Geometry: final body of the model. Coordinates: model frame, mm. Face numbers are marked on the shaded views. Give positions to 0.01 mm unless a question says otherwise; leave off trailing zeros. Write each loop counter-clockwise with the first axis right and the second up, starting at its lowest first coordinate (ties: lowest second). Pieces come first, ordered by that corner, then holes.
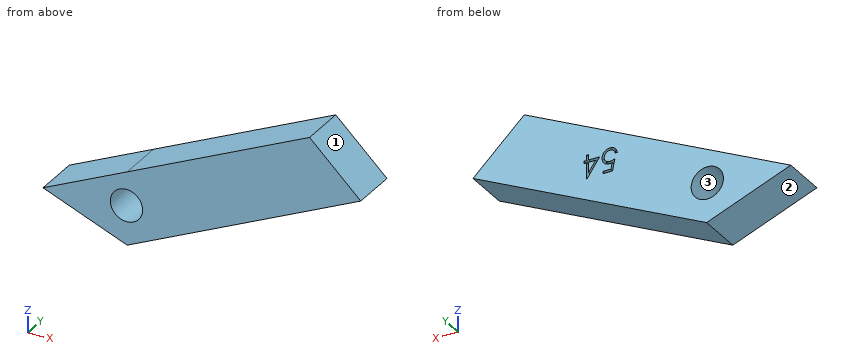
```python
from build123d import *

# Parameters (mm, degrees)
SKETCH1_R           = 2.2
BOSS_EXTRUDE1_DEPTH = 6.2
CUT_EXTRUDE1_DEPTH  = 1


with BuildPart() as part:
    # Sketch1 → Boss-Extrude1 (new body)
    with BuildSketch(Plane(origin=(0, 0, 0), x_dir=(-1, 0, 0), z_dir=(0, 1, 0))):
        Polygon((-127.443880814, 98.339887686), (-134.435779681, 91.672540756), (-102.538529649, 76.502840404), (-91.051660388, 81.032468444), (-102.547087364, 86.499465833), align=None)
        with Locations((-102.448365494, 81.883499702)):
            Circle(SKETCH1_R, mode=Mode.SUBTRACT)
    extrude(amount=BOSS_EXTRUDE1_DEPTH)

    # Sketch2 → Cut-Extrude1 (cut)
    with BuildSketch(Plane(origin=(0, 6.2, 0), x_dir=(1, 0, 0), z_dir=(0, 1, 0))):
        with BuildLine():
            Line((116.688123147, -87.22045081), (116.688123147, -87.546091836))
            Line((116.688123147, -87.546091836), (115.608165214, -87.546091836))
            Line((115.608165214, -87.546091836), (115.437076472, -88.381182982))
            add(Edge.make_bspline(
                [(115.437076472, -88.381182982), (115.470691444, -88.371902664), (115.535815135, -88.353923515), (115.631935866, -88.333961138), (115.723187365, -88.321927485), (115.782401451, -88.320284368), (115.811054838, -88.319489272)],
                knots=[0, 0, 0, 0, 0.000104595, 0.000202637, 0.000294305, 0.000380252, 0.000380252, 0.000380252, 0.000380252], degree=3))
            add(Edge.make_bspline(
                [(115.811054838, -88.319489272), (115.846509373, -88.320256656), (115.916221848, -88.321765526), (116.018220035, -88.336254275), (116.115586303, -88.359059769), (116.208117024, -88.3909191), (116.295983381, -88.431658643), (116.378376955, -88.482549303), (116.45653449, -88.541997397), (116.529053843, -88.610346086), (116.594843751, -88.685567839), (116.652688613, -88.766446764), (116.70182182, -88.852196858), (116.741337648, -88.94363741), (116.772892008, -89.039757499), (116.793894175, -89.141568485), (116.807879332, -89.248110708), (116.809441783, -89.320958425), (116.810238532, -89.358106059)],
                knots=[0, 0, 0, 0, 0.000106308, 0.000209029, 0.000308378, 0.000405929, 0.000502102, 0.000598312, 0.00069588, 0.000796219, 0.000896736, 0.000995218, 0.001094066, 0.001192613, 0.001293582, 0.001396995, 0.001504047, 0.001615439, 0.001615439, 0.001615439, 0.001615439], degree=3))
            add(Edge.make_bspline(
                [(116.810238532, -89.358106059), (116.809635213, -89.383979787), (116.80843673, -89.435377583), (116.802342011, -89.511708394), (116.790607469, -89.586423249), (116.774852462, -89.659532062), (116.754403269, -89.730896421), (116.729648198, -89.800720593), (116.69935323, -89.868569986), (116.66612334, -89.935086594), (116.628706892, -89.998766669), (116.587179246, -90.058319678), (116.543304836, -90.11463899), (116.496095865, -90.167120591), (116.445113534, -90.215419615), (116.390975278, -90.259822698), (116.334113097, -90.301080762), (116.27364727, -90.337519054), (116.210925161, -90.371049735), (116.145040992, -90.398557516), (116.0774945, -90.423150638), (116.007313506, -90.442753566), (115.934656976, -90.458113812), (115.859405144, -90.4685465), (115.781952679, -90.476145125), (115.729451774, -90.476620792), (115.702931841, -90.476861067)],
                knots=[0, 0, 0, 0, 7.7636e-05, 0.000154223, 0.000229512, 0.000304362, 0.000378447, 0.000452077, 0.000526407, 0.000601214, 0.00067506, 0.000747747, 0.00081887, 0.000889121, 0.000959302, 0.001029336, 0.001099058, 0.00116985, 0.001240974, 0.00131221, 0.00138383, 0.001456517, 0.001530612, 0.001606437, 0.001684346, 0.001763871, 0.001763871, 0.001763871, 0.001763871], degree=3))
            add(Edge.make_bspline(
                [(115.702931841, -90.476861067), (115.671295977, -90.476234378), (115.609056152, -90.475001442), (115.517869638, -90.462103245), (115.430135674, -90.443630263), (115.346560511, -90.41583879), (115.26639515, -90.38101603), (115.190718827, -90.337004931), (115.117597873, -90.28713103), (115.050004812, -90.228275281), (114.987270337, -90.163944627), (114.93111229, -90.094133052), (114.88109826, -90.019992773), (114.83802916, -89.941163733), (114.80129167, -89.857853066), (114.77243093, -89.769748629), (114.749136994, -89.677310768), (114.73928232, -89.613671513), (114.734276993, -89.581348246)],
                knots=[0, 0, 0, 0, 9.4843e-05, 0.000186593, 0.000275792, 0.000363484, 0.000450342, 0.000537514, 0.000625728, 0.000715478, 0.000805885, 0.000894984, 0.00098389, 0.001073836, 0.001164117, 0.001256635, 0.001351658, 0.001449737, 0.001449737, 0.001449737, 0.001449737], degree=3))
            Line((114.734276993, -89.581348246), (115.019212891, -89.581348246))
            add(Edge.make_bspline(
                [(115.019212891, -89.581348246), (115.026223796, -89.611625457), (115.039699146, -89.669819936), (115.069277218, -89.751581939), (115.105441262, -89.824442949), (115.148443778, -89.889366785), (115.199742735, -89.945980661), (115.258280145, -89.996433282), (115.323909866, -90.041949292), (115.396838009, -90.079888516), (115.473775589, -90.112245171), (115.554300129, -90.133791352), (115.636219072, -90.148941447), (115.691625879, -90.150457973), (115.719468299, -90.151220041)],
                knots=[0, 0, 0, 0, 9.3172e-05, 0.000179081, 0.000260145, 0.000336703, 0.000411917, 0.000488562, 0.000568128, 0.000650923, 0.00073478, 0.000817953, 0.000900557, 0.000983994, 0.000983994, 0.000983994, 0.000983994], degree=3))
            add(Edge.make_bspline(
                [(115.719468299, -90.151220041), (115.746644888, -90.150475478), (115.800155814, -90.149009428), (115.878906143, -90.137725467), (115.954936393, -90.120346813), (116.027496353, -90.094339159), (116.097855749, -90.062730021), (116.164234813, -90.02216706), (116.228553851, -89.975485472), (116.288813658, -89.922003386), (116.34400373, -89.863066591), (116.392768211, -89.80004067), (116.433387268, -89.732806102), (116.467617496, -89.662526885), (116.493610131, -89.588432765), (116.512153021, -89.510870985), (116.52304151, -89.429649967), (116.524539366, -89.374251379), (116.525302634, -89.346021724)],
                knots=[0, 0, 0, 0, 8.15e-05, 0.000160473, 0.000238226, 0.000315066, 0.000391338, 0.000469218, 0.000547964, 0.000629516, 0.000710512, 0.000789892, 0.000868102, 0.000945761, 0.001024012, 0.00110315, 0.001184644, 0.001269321, 0.001269321, 0.001269321, 0.001269321], degree=3))
            add(Edge.make_bspline(
                [(116.525302634, -89.346021724), (116.524705299, -89.320553006), (116.523536101, -89.270701615), (116.513983369, -89.19776805), (116.497367259, -89.128758933), (116.474304168, -89.06334102), (116.445022043, -89.001452612), (116.409238602, -88.943029836), (116.366282306, -88.888842716), (116.317213235, -88.838865899), (116.263457727, -88.792742334), (116.204090903, -88.753423056), (116.140355112, -88.720345073), (116.073018261, -88.691799103), (116.000478675, -88.671296999), (115.924172873, -88.655904703), (115.843276859, -88.647000766), (115.787967735, -88.645765339), (115.75953741, -88.645130297)],
                knots=[0, 0, 0, 0, 7.6388e-05, 0.000149519, 0.000220172, 0.000288967, 0.000357247, 0.000425206, 0.000494043, 0.000564207, 0.000635056, 0.000706145, 0.000777268, 0.000850264, 0.000925136, 0.001002969, 0.001083601, 0.001168886, 0.001168886, 0.001168886, 0.001168886], degree=3))
            add(Edge.make_bspline(
                [(115.75953741, -88.645130297), (115.734927596, -88.645656977), (115.684114573, -88.646744435), (115.606170295, -88.654751329), (115.524262803, -88.667668403), (115.438706082, -88.685435928), (115.349243193, -88.708686976), (115.256062929, -88.736549416), (115.158969373, -88.769861515), (115.093548295, -88.795018594), (115.059918019, -88.80795081)],
                knots=[0, 0, 0, 0, 7.3822e-05, 0.000152423, 0.000234822, 0.000322511, 0.00041445, 0.000512043, 0.000614219, 0.000722306, 0.000722306, 0.000722306, 0.000722306], degree=3))
            Line((115.059918019, -88.80795081), (115.385559044, -87.22045081))
            Line((115.385559044, -87.22045081), (116.688123147, -87.22045081))
        make_face()
        Polygon((118.869027594, -87.139040554), (118.926905198, -87.139040554), (118.926905198, -89.337117477), (119.293251352, -89.337117477), (119.293251352, -89.662758503), (118.926905198, -89.662758503), (118.926905198, -90.39545081), (118.641969301, -90.39545081), (118.641969301, -89.662758503), (117.135879557, -89.662758503), align=None)
        Polygon((118.641969301, -89.337117477), (118.641969301, -87.958231259), (117.69557507, -89.337117477), align=None, mode=Mode.SUBTRACT)
    extrude(amount=-CUT_EXTRUDE1_DEPTH, mode=Mode.SUBTRACT)


solid = part.part
```
Item 1: Section C-C, the plane x = 95. Return the cut outline in (y, z), plus the area to 3 significant figures.
Found:
outline: (0, 79.48) - (6.2, 79.48) - (6.2, 82.91) - (0, 82.91) - close
area: 21.3 mm2
Item 2: Section B-B, the plane y = 4.5. Return the cut outline in (x, z).
Found:
outline: (91.05, 81.03) - (102.54, 76.5) - (134.44, 91.67) - (127.44, 98.34) - close; hole circle Ø4.4 at (102.45, 81.88)
Item 3: Section A-A, the plane z = 83. Return the cut outline in (x, y).
Found:
outline: (95.19, 0) - (100.55, 0) - (100.55, 6.2) - (95.19, 6.2) - close; (104.34, 0) - (116.2, 0) - (116.2, 6.2) - (104.34, 6.2) - close
Item 4: Section D-D, the plane z = 80.25. Return the cut outline in (x, y), plus the area to 3 significant figures.
Found:
outline: (93.04, 0) - (100.97, 0) - (100.97, 6.2) - (93.04, 6.2) - close; (103.92, 0) - (110.42, 0) - (110.42, 6.2) - (103.92, 6.2) - close
area: 89.5 mm2
Item 5: Pull-direction query (X, two-part tool) for the marked faces 1, 2 and 3; classes: +X half, -X half, draft (parallel to the pull), parting line (faces both ways), or undercut.
Found:
face 1: +X half
face 2: -X half
face 3: undercut
Item 6: Pin query (flat end, axial travel): pin 1 Ø0.5 at (x, y) = (116, 6) entering from +Z; pin 2 Ø1.5 at (y, z) = (2, 81) entering from +X; pin 3 Ø0.8 at (y, z) = (5.5, 88.5) entering from -X. Return the tip coordinate at first contact, or that it passes through.
Found:
pin 1: stops at z = 93.02
pin 2: stops at x = 113.57
pin 3: stops at x = 105.91
Item 7: Line query: L1, parallel to Y at x = 116, z = 90.25; L2, parallel to Z at x = 104, y = 2.25; L3, parallel to Z at x = 102, y = 3.5. Output: solid intervals per line, ascending.
Found:
L1: y = 0 to 5.2
L2: z = 77.2 to 80.32, 83.44 to 87.19
L3: z = 76.72 to 79.73, 84.04 to 86.24
